Source: three-view drawing plus pictorial views. Frame: mm from the lowest corner of the part. A direction names the side the tool comes from. Round coordinates to 2 decimals unless told otherwise and drop trailing zeros. Write each loop counter-clockwise with the first axis right and the second up, starting at its lowest first coordinate (ties: lowest second). Pieces come first, ordered by that corner, then holes. Notation, with made-up numbers: M -39.75,-18 L -18.75,-18 A35 cw -18.75,19 Z; hole C -39,68.5 d6. An arc over 180 degrees is marked long. Put each result on its own line as item: value. Start each with the question number.
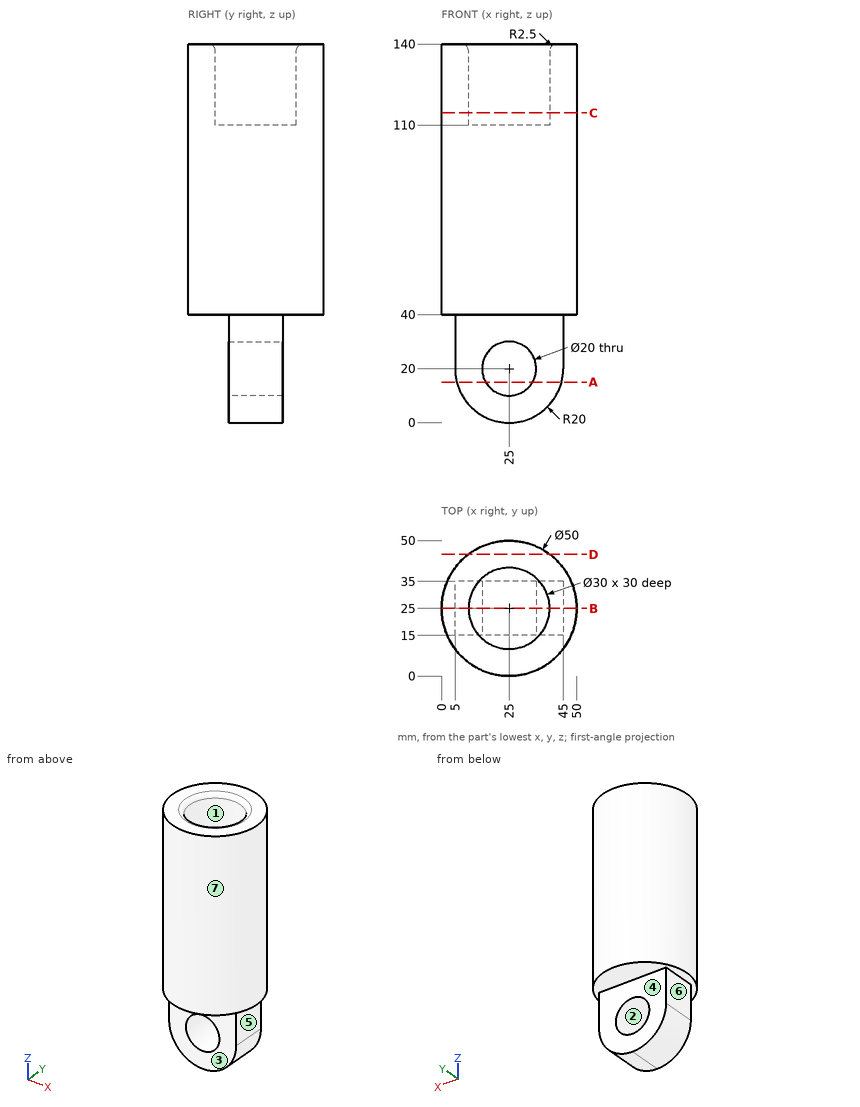
(1) Access query for the marked faces 5, 6 and 7. Directions: +Z, -Z, +X, -X, +Y, -Y. A direction counts if a zero-diameter tool reaches every point of the face in a straight line with its end or side. Return the directions, or none.
(2) Section query C-C (z = 114.5). Return loops of the section in (x, y).
(3) Section query D-D (y = 45). Return loops of the section in (x, z), and give its area (3 significant figures).
(4) Ray query, line 1 along X through (y, z) = (24, 20); line 2 along Z through (x, y) = (25, 22.5); line 3 along Y through (x, z) = (25, 124). Return the intervals inside material, ascending.
(5) Section query B-B (y = 25). Return loops of the section in (x, z), and give its area (3 significant figures).
(6) Section query A-A (z = 15). Return loops of the section in (x, y), and give its area (3 significant figures).
(7) Contact query for flat-ended pins moving along their axis: P1, Ø5, axis at y = 38.5, z = 118.5, coming from the +X side; P2, Ø12, axis at x = 18, z = 21.5, coming from the +Y side; P3, Ø2, axis at x = 30, y = 37.5, coming from the -Z side. Output: stop coordinate, or through.
(8) Pull-direction query (Y, two-part tool) for the marked faces 1, 2, 3 and 4; classes: +Y half, -Y half, draft (parallel to the pull), parting line (faces both ways), or undercut.
Entries:
1. face 5: -Z, +X, +Y, -Y
1. face 6: -Z, -X, +Y, -Y
1. face 7: +Z, -Z
2. outline: C 25,25 d50; hole C 25,25 d30
3. outline: M 10,40 L 40,40 L 40,140 L 10,140 Z
3. area: 3,000 mm2
4. line 1: 5 to 15, 35 to 45
4. line 2: 0 to 10, 30 to 110
4. line 3: 0 to 10, 40 to 50
5. outline: M 0,40 L 5,40 L 5,20 A20 ccw 45,20 L 45,40 L 50,40 L 50,140 L 42.5,140 A2.5 ccw 40,137.5 L 40,110 L 10,110 L 10,137.5 A2.5 ccw 7.5,140 L 0,140 Z; hole C 25,20 d20
5. area: 5,210 mm2
6. outline: M 5.64,15 L 16.34,15 L 16.34,35 L 5.64,35 Z; M 33.66,15 L 44.36,15 L 44.36,35 L 33.66,35 Z
6. area: 428 mm2
7. P1: x = 47.45
7. P2: y = 35
7. P3: z = 40
8. face 1: undercut
8. face 2: draft
8. face 3: -Y half
8. face 4: +Y half
